from build123d import *

# Parameters (mm, degrees)
CROQUIS1_R              = 25
CROQUIS1_W              = 10.3
CROQUIS1_H              = 5
CROQUIS1_R_2            = 1.15
SALIENTE_EXTRUIR1_DEPTH = 2
REDONDEO1_R             = 1
CROQUIS2_R              = 20
CORTAR_EXTRUIR1_DEPTH   = 1


with BuildPart() as part:
    # Croquis1 → Saliente-Extruir1 (new body)
    # profile 1 of 3: a face of its own
    with BuildSketch(Plane(origin=(0, 0, 0), x_dir=(1, 0, 0), z_dir=(0, 1, 0))):
        Circle(CROQUIS1_R)
    # profile 2 of 3: a face of its own
    with BuildSketch(Plane(origin=(0, 0, 0), x_dir=(1, 0, 0), z_dir=(0, 1, 0))):
        with Locations((25, 0)):
            Rectangle(CROQUIS1_W, CROQUIS1_H)
        with Locations(Location((27.575, 0, 0), (0, 0, 270))):
            Circle(CROQUIS1_R_2, mode=Mode.SUBTRACT)
    # profile 3 of 3: a face of its own
    with BuildSketch(Plane(origin=(0, 0, 0), x_dir=(1, 0, 0), z_dir=(0, 1, 0))):
        with Locations((-25, 0)):
            Rectangle(CROQUIS1_W, CROQUIS1_H)
        with Locations(Location((-27.575, 0, 0), (0, 0, 270))):
            Circle(CROQUIS1_R_2, mode=Mode.SUBTRACT)
    extrude(amount=SALIENTE_EXTRUIR1_DEPTH)

    # Redondeo1
    redondeo1_edges = [part.edges().sort_by_distance(p)[0] for p in [
        (24.874685928, 1, -2.5),
        (24.874685928, 1, 2.5),
    ]]
    fillet(redondeo1_edges, radius=REDONDEO1_R)

    # Croquis2 → Cortar-Extruir1 (cut)
    with BuildSketch(Plane(origin=(0, 2, 0), x_dir=(1, 0, 0), z_dir=(0, 1, 0))):
        with Locations(Location((0, 0, 0), (0, 0, 270))):
            Circle(CROQUIS2_R)
    extrude(amount=-CORTAR_EXTRUIR1_DEPTH, mode=Mode.SUBTRACT)


solid = part.part
Design review of the part built by this model. Coordinates are the model's own, in mm. A direction names the side the tool comes from. Round coordinates to 2 decimals unless told otherwise and drop trailing zeros. Loops run counter-clockwise (first coordinate to the right, second up) from the corner with the lowest first, then second, coordinate; pieces in that order, holes last. Notation, with made-up numbers: (29, 51) -> (49, 51) arc R16 cw to (49, 57) -> close; hole circle Ø11 at (62, 47.5). An arc over 180 degrees is marked (long way). Use one line per item in the form item = value. Start each with the question number.
Q1. We need section C-C on x = 0. Give the boundary of the cut face in (y, z).
Q2. We need section A-A on z = 0. Give the boundary of the cut face in (x, y) (3 decimals), then the cut area to 3 significant figures.
Q3. Machinability: for faces 1 (the face through (-28, 1, 2.5)), 2 (the face through (28, 1, -2.5)), 3 (the face through (-28, 1, -2.5)), 4 (the face through (0, 1, 0)), which of the approach directions +Z, -Z, +X, -X, +Y, -Y give a long, thin tool a straight path to every point of the face, cutting with its end or side? Answer none if there is none.
Q4. We need section B-B on y = 0.45. Give the boundary of the cut face in (x, z) (3 decimals).
Q5. Draft analysis for pull direction X (two halves, no side actions). For faces 5 (the face through (0, 0, 0)), 6 (the face through (-30.15, 1, 0)), 7 (the face through (-19.524, 1.507, -4.336)), state which applies: +X half, -X half, draft (parallel to the pull), parting line (faces both ways), or undercut.
Q6. Wall thickness on line 1 along X through (y, z) = (0.4, 0) (3 decimals); line 2 along X through (y, z) = (1.6, 0) (3 decimals); line 3 along Y through (x, z) = (0, 15.5): over which ranges is each line inside the solid? List them lowest first. Write a range as [from, to].
Q7. We need section D-D on z = 15.5. Give the boundary of the cut face in (x, y), then the cut area to 3 significant figures.
Q8. For pin 1 Ø0.6 at (x, y) = (27.5, 1) entering from +Z; pin 2 Ø0.6 at (x, y) = (-28.5, 0.5) entering from -Z; pin 3 Ø1 at (y, z) = (1, 13) entering from +X, all flat-tipped, find the tip position at first contact; note any pin that passes through.
Calculated:
q1.outline = (0, -25) -> (2, -25) -> (2, -20) -> (1, -20) -> (1, 20) -> (2, 20) -> (2, 25) -> (0, 25) -> close
q2.outline = (-30.15, 0) -> (-28.725, 0) -> (-28.725, 2) -> (-30.15, 2) -> close; (-26.425, 0) -> (26.425, 0) -> (26.425, 2) -> (20, 2) -> (20, 1) -> (-20, 1) -> (-20, 2) -> (-26.425, 2) -> close; (28.725, 0) -> (30.15, 0) -> (30.15, 2) -> (28.725, 2) -> close
q2.area = 71.4 mm²
q3.face_1 = +Z, -X, +Y, -Y
q3.face_2 = -Z, +X, +Y, -Y
q3.face_3 = -Z, -X, +Y, -Y
q3.face_4 = +Y
q4.outline = (-30.15, -2.5) -> (-24.875, -2.5) arc R25 ccw to (24.772, -3.365) arc R1 cw to (25.763, -2.5) -> (30.15, -2.5) -> (30.15, 2.5) -> (25.763, 2.5) arc R1 cw to (24.772, 3.365) arc R25 ccw to (-24.875, 2.5) -> (-30.15, 2.5) -> close; hole circle Ø2.3 at (-27.575, 0); hole circle Ø2.3 at (27.575, 0)
q5.face_5 = draft
q5.face_6 = -X half
q5.face_7 = undercut
q6.line_1 = [-30.15, -28.725], [-26.425, 26.425], [28.725, 30.15]
q6.line_2 = [-30.15, -28.725], [-26.425, -20], [20, 26.425], [28.725, 30.15]
q6.line_3 = [0, 1]
q7.outline = (-19.62, 0) -> (19.62, 0) -> (19.62, 2) -> (12.64, 2) -> (12.64, 1) -> (-12.64, 1) -> (-12.64, 2) -> (-19.62, 2) -> close
q7.area = 53.2 mm²
q8.pin_1 = 2.5
q8.pin_2 = -2.5
q8.pin_3 = 21.65
